Can you work these out from the model? Positions are in its coordinate system, mm. A direction names the side the tool comes from. Round coordinates to 2 decimals unless told otherwise and drop trailing zeros. Return JSON: item names as keys, results as strings.
```python
from build123d import *

# Parameters (mm, degrees)
SZKIC1_R                    = 4
SZKIC1_W                    = 7.071067812
SZKIC1_H                    = 7.071067812
DODANIE_WYCI_GNI_CIE1_DEPTH = 500


with BuildPart() as part:
    # Szkic1 → Dodanie-wyciągnięcie1 (new body)
    with BuildSketch(Plane.XY):
        with BuildLine():
            Line((4, 20), (4, 15.5))
            Line((4, 15.5), (6.166140933, 15.5))
            Line((6.166140933, 15.5), (6.166140933, 17.75))
            ThreePointArc((6.166140933, 17.75), (7.757131191, 17.090990258), (8.416140933, 15.5))
            ThreePointArc((8.416140933, 15.5), (7.228277524, 11.189149476), (4, 8.095175343))
            Line((4, 8.095175343), (-4, 8.095175343))
            ThreePointArc((-4, 8.095175343), (-7.228277524, 11.189149476), (-8.416140933, 15.5))
            ThreePointArc((-8.416140933, 15.5), (-7.757131191, 17.090990258), (-6.166140933, 17.75))
            Line((-6.166140933, 17.75), (-6.166140933, 15.5))
            Line((-6.166140933, 15.5), (-4, 15.5))
            Line((-4, 15.5), (-4, 20))
            Line((-4, 20), (-19, 20))
            ThreePointArc((-19, 20), (-19.707106781, 19.707106781), (-20, 19))
            Line((-20, 19), (-20, 4))
            Line((-20, 4), (-15.5, 4))
            Line((-15.5, 4), (-15.5, 6.166140933))
            Line((-15.5, 6.166140933), (-17.75, 6.166140933))
            ThreePointArc((-17.75, 6.166140933), (-17.090990258, 7.757131191), (-15.5, 8.416140933))
            ThreePointArc((-15.5, 8.416140933), (-11.189149476, 7.228277524), (-8.095175343, 4))
            Line((-8.095175343, 4), (-8.095175343, -4))
            ThreePointArc((-8.095175343, -4), (-11.189149476, -7.228277524), (-15.5, -8.416140933))
            ThreePointArc((-15.5, -8.416140933), (-17.090990258, -7.757131191), (-17.75, -6.166140933))
            Line((-17.75, -6.166140933), (-15.5, -6.166140933))
            Line((-15.5, -6.166140933), (-15.5, -4))
            Line((-15.5, -4), (-20, -4))
            Line((-20, -4), (-20, -19))
            ThreePointArc((-20, -19), (-19.707106781, -19.707106781), (-19, -20))
            Line((-19, -20), (-4, -20))
            Line((-4, -20), (-4, -15.5))
            Line((-4, -15.5), (-6.166140933, -15.5))
            Line((-6.166140933, -15.5), (-6.166140933, -17.75))
            ThreePointArc((-6.166140933, -17.75), (-7.757131191, -17.090990258), (-8.416140933, -15.5))
            ThreePointArc((-8.416140933, -15.5), (-7.228277524, -11.189149476), (-4, -8.095175343))
            Line((-4, -8.095175343), (4, -8.095175343))
            ThreePointArc((4, -8.095175343), (7.228277524, -11.189149476), (8.416140933, -15.5))
            ThreePointArc((8.416140933, -15.5), (7.757131191, -17.090990258), (6.166140933, -17.75))
            Line((6.166140933, -17.75), (6.166140933, -15.5))
            Line((6.166140933, -15.5), (4, -15.5))
            Line((4, -15.5), (4, -20))
            Line((4, -20), (19, -20))
            ThreePointArc((19, -20), (19.707106781, -19.707106781), (20, -19))
            Line((20, -19), (20, -4))
            Line((20, -4), (15.5, -4))
            Line((15.5, -4), (15.5, -6.166140933))
            Line((15.5, -6.166140933), (17.75, -6.166140933))
            ThreePointArc((17.75, -6.166140933), (17.090990258, -7.757131191), (15.5, -8.416140933))
            ThreePointArc((15.5, -8.416140933), (11.189149476, -7.228277524), (8.095175343, -4))
            Line((8.095175343, -4), (8.095175343, 4))
            ThreePointArc((8.095175343, 4), (11.189149476, 7.228277524), (15.5, 8.416140933))
            ThreePointArc((15.5, 8.416140933), (17.090990258, 7.757131191), (17.75, 6.166140933))
            Line((17.75, 6.166140933), (15.5, 6.166140933))
            Line((15.5, 6.166140933), (15.5, 4))
            Line((15.5, 4), (20, 4))
            Line((20, 4), (20, 19))
            ThreePointArc((20, 19), (19.707106781, 19.707106781), (19, 20))
            Line((19, 20), (4, 20))
        make_face()
        Circle(SZKIC1_R, mode=Mode.SUBTRACT)
        with Locations((-14.214466094, 14.214466094)):
            Rectangle(SZKIC1_W, SZKIC1_H, mode=Mode.SUBTRACT)
        with Locations((14.214466094, 14.214466094)):
            Rectangle(SZKIC1_W, SZKIC1_H, mode=Mode.SUBTRACT)
        with Locations((14.214466094, -14.214466094)):
            Rectangle(SZKIC1_W, SZKIC1_H, mode=Mode.SUBTRACT)
        with Locations((-14.214466094, -14.214466094)):
            Rectangle(SZKIC1_W, SZKIC1_H, mode=Mode.SUBTRACT)
    extrude(amount=DODANIE_WYCI_GNI_CIE1_DEPTH)


solid = part.part
```
Q1. If I drill on line 1 along X through (y, z) = (13.5, 386.5); line 2 along Y through (x, z) = (-16, 102); line 3 along Y through (x, z) = (0, 275), over which ranges is the centre line in solid material (lowest first)?
Results:
{"line 1": "x = -20 to -17.75, -10.68 to -8.18, 8.18 to 10.68, 17.75 to 20", "line 2": "y = -20 to -17.75, -10.68 to -8.36, -6.17 to -4, 4 to 6.17, 8.36 to 10.68, 17.75 to 20", "line 3": "y = -8.1 to -4, 4 to 8.1"}
Q2. Thinking about a two-plate mould opening in X: for faces 4 (the flat face through (0, 8.095, 246)), 5 (the flat face through (-5, 0, 0)), 6 (the flat face through (20, 11, 246)), 7 (the flat face through (-8.095, 0, 246)), which applies, pulls with the +X half, pulls with the -X half, needs draft (parallel to the pull), parting line crosses it, or undercut?
Results:
{"face 4": "undercut", "face 5": "needs draft", "face 6": "pulls with the +X half", "face 7": "pulls with the -X half"}
Q3. Suppose I cut it at A-A, the plane z = 368. State how many separate pieces and enclosed holes the cut face has, plus the area to 3 significant figures.
Results:
{"separate pieces": "1", "enclosed holes": "5", "area": "750 mm2"}
Q4. On a 3-axis mill with a long thin cutter (end or side, diameter ignored), from which of +Z, -Z, +X, -X, +Y, -Y can I reach the whole of each face in a straight line? I mean faces 1 (the flat face through (0, -8.095, 246)), 2 (the flat face through (8.095, 0, 246)), 3 (the flat face through (-11, 20, 246)). Say none if no direction works.
Results:
{"face 1": "+Z, -Z, -Y", "face 2": "+Z, -Z, +X", "face 3": "+Z, -Z, +X, -X, +Y"}
Q5. I'm going to push a flat-ended pin straight in: pin 1 Ø3 at (y, z) = (1, 117.5) entering from -X. Where does the tip first touch, or does it pass through?
Results:
{"pin 1": "stops at x = -8.1"}
